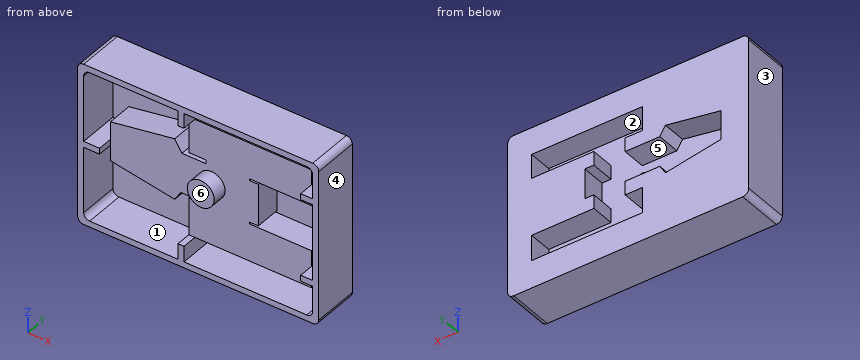
from build123d import *

# Parameters (mm, degrees)
SKETCH1_W           = 84.5
SKETCH1_H           = 54
BOSS_EXTRUDE2_DEPTH = 15.5
FILLET1_R           = 2
Y_WING_START        = -26.76167351
Y_WING_DEPTH        = 8
Y_WING_START_2      = -32.76167351
Y_WING_2_OUTLINE_R  = 2.5
Y_WING_2_DEPTH      = 6
SKETCH2_W           = 80.5
SKETCH2_H           = 50
CUT_EXTRUDE1_DEPTH  = 13.5
SKETCH3_W           = 2.008539682
SKETCH3_H           = 5.255332567
SKETCH3_H_2         = 4.996733938
BOSS_EXTRUDE3_DEPTH = 13.5
SKETCH4_R           = 4.5
CUT_EXTRUDE2_DEPTH  = 5
SKETCH5_W           = 2
SKETCH5_H           = 54
CUT_EXTRUDE3_DEPTH  = 15.5
SKETCH6_W           = 2
SKETCH6_H           = 50
BOSS_EXTRUDE4_DEPTH = 13.5
FILLET2_R           = 2


with BuildPart() as part:
    # Sketch1 → Boss-Extrude2 (new body)
    with BuildSketch(Plane(origin=(0, 0, 0), x_dir=(1, 0, 0), z_dir=(0, 1, 0))):
        with Locations((42.25, 27)):
            Rectangle(SKETCH1_W, SKETCH1_H)
    extrude(amount=BOSS_EXTRUDE2_DEPTH)

    # Fillet1
    fillet1_edges = [part.edges().sort_by_distance(p)[0] for p in [
        (0, 7.75, -54),
        (84.5, 7.75, -54),
        (84.5, 7.75, 0),
        (0, 7.75, 0),
    ]]
    fillet(fillet1_edges, radius=FILLET1_R)


with BuildPart() as body_2:
    # Y-Wing: read off the stored shape, not the designer's step
    # Y-Wing outline → Y-Wing (new body)
    with BuildSketch(Plane(origin=(0, 0, 0), x_dir=(1, 0, 0), z_dir=(0, 1, 0)).offset(Y_WING_START)):
        Polygon((-37.998848216, 80.77793428), (-49.561243891, 80.77793428), (-51.452110178, 83.77793428), (-69.950345376, 80.625586413), (-69.950345376, 70.93293428), (-51.452110178, 67.77793428), (-49.561243891, 70.77793428), (-37.998848216, 70.77793428), (-37.998848216, 66.17793428), (-43.764531914, 66.17793428), (-43.764531914, 58.130000785), (-6.764531914, 58.130000785), (-6.764531914, 66.17793428), (-27.548546514, 66.17793428), (-27.548546514, 70.77793428), (-24.545586254, 70.77793428), (-24.545586254, 80.77793428), (-27.548546514, 80.77793428), (-27.548546514, 85.37793428), (-6.764531914, 85.37793428), (-6.764531914, 93.87793428), (-43.764531914, 93.87793428), (-43.764531914, 85.37793428), (-37.998848216, 85.37793428), align=None)
    extrude(amount=Y_WING_DEPTH)

    # Y-Wing 2 outline → Y-Wing 2 (add)
    with BuildSketch(Plane(origin=(0, 0, 0), x_dir=(1, 0, 0), z_dir=(0, 1, 0)).offset(Y_WING_START_2)):
        with Locations((-38.150345376, 75.778331613)):
            Circle(Y_WING_2_OUTLINE_R)
    extrude(amount=Y_WING_2_DEPTH)


with BuildPart() as body_2_1:
    # Body-Move/Copy3: moved
    add(body_2.part.moved(Location((81.260162004, 34.341820547, 49.133266847))))


with BuildPart() as part_1:
    add(part.part)

    # Intersect1: read off the stored shape, not the designer's step
    # Intersect1: cut body 2
    add(body_2_1.part, mode=Mode.SUBTRACT)

    # Sketch2 → Cut-Extrude1 (cut)
    with BuildSketch(Plane.XZ):
        with Locations((42.25, -27)):
            Rectangle(SKETCH2_W, SKETCH2_H)
        Polygon((30.788040431, -16.448642605), (33.204506118, -20.282545146), (41.261313787, -20.282545146), (41.261313787, -19.044667433), (35.495630089, -19.044667433), (35.495630089, -6.996733938), (76.495630089, -6.996733938), (76.495630089, -19.044667433), (55.71161549, -19.044667433), (55.71161549, -19.644667433), (58.714575749, -19.644667433), (58.714575749, -33.644667433), (55.71161549, -33.644667433), (55.71161549, -34.244667433), (76.495630089, -34.244667433), (76.495630089, -46.744667433), (35.495630089, -46.744667433), (35.495630089, -34.244667433), (41.261313787, -34.244667433), (41.261313787, -33.644667433), (36.074948333, -33.644667433), (32.802458964, -33.644667433), (30.788147827, -36.840521868), (9.309816627, -33.180325595), (9.309816627, -20.111899958), align=None, mode=Mode.SUBTRACT)
    extrude(amount=-CUT_EXTRUDE1_DEPTH, mode=Mode.SUBTRACT)

    # Sketch3 → Boss-Extrude3 (add)
    with BuildSketch(Plane.XZ.offset(-13.5)):
        Polygon((2, -27), (2, -28.000523913), (9.309816627, -28.000523913), (9.309816627, -27), (9.309816627, -26.003783182), (2, -26.003783182), align=None)
        with Locations((36.49989993, -49.372333717)):
            Rectangle(SKETCH3_W, SKETCH3_H)
        Polygon((76.495630089, -40.494667433), (76.495630089, -39.49850229), (82.5, -39.49850229), (82.5, -40.494667433), (82.5, -41.494277076), (76.495630089, -41.494277076), align=None)
        Polygon((76.495630089, -13.020700685), (76.495630089, -14.018243481), (82.5, -14.018243481), (82.5, -13.020700685), (82.5, -12.020776308), (76.495630089, -12.020776308), align=None)
        with Locations((36.49989993, -4.498366969)):
            Rectangle(SKETCH3_W, SKETCH3_H_2)
    extrude(amount=BOSS_EXTRUDE3_DEPTH)

    # Sketch4 → Cut-Extrude2 (cut)
    with BuildSketch(Plane.XZ):
        Polygon((9.309816627, -20.111899958), (30.788040431, -16.448642605), (33.204506118, -20.282545146), (41.261313787, -20.282545146), (41.261313787, -19.044667433), (35.495630089, -19.044667433), (35.495630089, -6.996733938), (76.495630089, -6.996733938), (76.495630089, -19.044667433), (55.71161549, -19.044667433), (55.71161549, -19.644667433), (58.714575749, -19.644667433), (58.714575749, -33.644667433), (55.71161549, -33.644667433), (55.71161549, -34.244667433), (76.495630089, -34.244667433), (76.495630089, -46.744667433), (35.495630089, -46.744667433), (35.495630089, -34.244667433), (41.261313787, -34.244667433), (41.261313787, -33.644667433), (32.802458964, -33.644667433), (30.788147827, -36.840521868), (9.309816627, -33.180325595), align=None)
        with Locations(Location((43.109816627, -26.645064766, 0), (0, 0, 270))):
            Circle(SKETCH4_R, mode=Mode.SUBTRACT)
    extrude(amount=-CUT_EXTRUDE2_DEPTH, mode=Mode.SUBTRACT)

    # Sketch5 → Cut-Extrude3 (cut)
    with BuildSketch(Plane(origin=(0, 0, 0), x_dir=(-1, 0, 0), z_dir=(0, -1, 0))):
        with Locations((-1, 27)):
            Rectangle(SKETCH5_W, SKETCH5_H)
        with Locations((-83.5, 27)):
            Rectangle(SKETCH5_W, SKETCH5_H)
    extrude(amount=-CUT_EXTRUDE3_DEPTH, mode=Mode.SUBTRACT)

    # Sketch6 → Boss-Extrude4 (add)
    with BuildSketch(Plane(origin=(0, 13.5, 0), x_dir=(-1, 0, 0), z_dir=(0, -1, 0))):
        with Locations((-3, 27)):
            Rectangle(SKETCH6_W, SKETCH6_H)
        with Locations((-81.5, 27)):
            Rectangle(SKETCH6_W, SKETCH6_H)
    extrude(amount=BOSS_EXTRUDE4_DEPTH)

    # Fillet2
    fillet2_edges = [part_1.edges().sort_by_distance(p)[0] for p in [
        (82.5, 7.75, -54),
        (2, 7.75, -54),
        (82.5, 7.75, 0),
        (2, 7.75, 0),
        (4, 6.75, -52),
        (4, 6.75, -2),
        (80.5, 6.75, -2),
        (80.5, 6.75, -52),
    ]]
    fillet(fillet2_edges, radius=FILLET2_R)


solid = part_1.part
Design review of the part built by this model. Coordinates are the model's own, in mm. Face numbers are marked on the shaded views. A direction names the side the tool comes from. Give positions to 0.01 mm unless a question says otherwise; leave off trailing zeros. Loops run counter-clockwise (first coordinate to the right, second up) from the corner with the lowest first, then second, coordinate; pieces in that order, holes last. Notation, with made-up numbers: (-23.75, 56.5) -> (31.25, 56.5) arc R9 ccw to (31.25, 72.5) -> close; hole circle Ø11 at (3, 17.25). An arc over 180 degrees is marked (long way). One line per question, with ' | ' between items. Start each with the question number.
(1) We need section D-D (x = 12.5). State the section outline as (y, z) points.
(2) We need section A-A (x = 61). State the section outline as (y, z) points.
(3) We need section B-B (z = -15.5). State the section outline as (x, y) points.
(4) Draft analysis for pull direction X (two halves, no side actions). For the marked faces 4, 5 and 6, state which applies: +X half, -X half, draft (parallel to the pull), parting line (faces both ways), or undercut.
(5) For the marked faces 1, 2 and 3, list the 3-axis set-ups (+Z, -Z, +X, -X, +Y, -Y) from which the entire face can be reached by the end or side of a thin tool; tool diameter is ignored.
(6) Insertion check: P1, Ø3, axis at x = 51.5, z = -25.5, coming from the -Y side; P2, Ø1.5, axis at x = 20.5, z = -14, coming from the -Y side; P3, Ø4, axis at x = 44, z = -26.5, coming from the +Y side. Each pin has a flat end and moves straight along its axis. Give the tip position at first contact, or say it passes through.
(7) For line 1 (Z direction, x = 7, y = 11.75); line 2 (X direction, y = 11, z = -11.5); line 3 (Z direction, x = 48, y = 11), list the stretches that pass through material, from the lowest coordinate up.
(8) We need section C-C (y = 11.75). State how many separate pieces and enclosed holes the cut face has, and give its area (3 significant figures).
The answers:
1) outline: (0, -54) -> (15.5, -54) -> (15.5, -31.7) -> (7.58, -31.7) -> (7.58, -21.6) -> (15.5, -21.6) -> (15.5, 0) -> (0, 0) -> (0, -2) -> (13.5, -2) -> (13.5, -19.57) -> (5, -19.57) -> (5, -33.72) -> (13.5, -33.72) -> (13.5, -52) -> (0, -52) -> close
2) outline: (0, -54) -> (15.5, -54) -> (15.5, -44.74) -> (7.58, -44.74) -> (7.58, -36.24) -> (15.5, -36.24) -> (15.5, -17.04) -> (7.58, -17.04) -> (7.58, -9) -> (15.5, -9) -> (15.5, 0) -> (0, 0) -> (0, -2) -> (13.5, -2) -> (13.5, -7) -> (5, -7) -> (5, -19.04) -> (13.5, -19.04) -> (13.5, -34.24) -> (5, -34.24) -> (5, -46.74) -> (13.5, -46.74) -> (13.5, -52) -> (0, -52) -> close
3) outline: (2, 0) -> (4, 0) -> (4, 13.5) -> (35.5, 13.5) -> (35.5, 5) -> (76.5, 5) -> (76.5, 13.5) -> (80.5, 13.5) -> (80.5, 0) -> (82.5, 0) -> (82.5, 15.5) -> (74.5, 15.5) -> (74.5, 7.58) -> (37.5, 7.58) -> (37.5, 15.5) -> (2, 15.5) -> close
4) face 4: +X half | face 5: undercut | face 6: draft
5) face 1: -Y | face 2: +Y | face 3: +Z, -Z, -X, +Y, -Y
6) P1: stops at y = 5 | P2: stops at y = 13.5 | P3: stops at y = 7.58
7) line 1: z = -54 to -52, -28 to -26, -2 to 0 | line 2: x = 2 to 4, 35.5 to 37.5, 74.5 to 76.5, 80.5 to 82.5 | line 3: z = -54 to -52, -46.74 to -44.74, -9 to -7, -2 to 0
8) separate pieces: 1 | enclosed holes: 6 | area: 1,120 mm^2
